Source: CAD feature listing. Evaluate the final solid. Frame: model axes, mm. A direction names the side the tool comes from. Round coordinates to 2 decimals unless told otherwise and drop trailing zeros. Loops run counter-clockwise (first coordinate to the right, second up) from the corner with the lowest first, then second, coordinate; pieces in that order, holes last. Notation, with made-up numbers: M -8,12 L 34,12 A16 ccw 34,43 Z; hole C -6.75,23 d10. An arc over 180 degrees is marked long. Write each question's results on one line, items separated by ' | '. Start each with the question number.
1. Set-up query: faces 5 (the flat face through (-12, 108, -20)), 6 (the flat face through (0, 125, -10)), 7 (the flat face through (10, 1, -124)). Return all of +Z, -Z, +X, -X, +Y, -Y with unobstructed straight access to the full face (end or side cutting, diameter ignored); none if empty.
2. Section C-C on x = -5. Output: boundary loops of the cut face in (y, z), and give its area (3 significant figures).
3. Section A-A on z = -42.5. Output: boundary loops of the cut face in (x, y).
4. Section B-B on y = -23. Output: boundary loops of the cut face in (x, z).
5. Ray query, line 1 (Y direction, x = 1, z = -21.5); line 2 (Z direction, x = -3.75, y = -42); line 3 (Z direction, x = 1.5, y = 52.5). Return the intervals inside material, ascending.
6. Contact query for flat-ended pins moving along their axis: pin 1 Ø22 at (y, z) = (9.5, -0.5) entering from -X; pin 2 Ø12 at (x, z) = (0.5, -51) entering from +Y; pin 3 Ø5.5 at (x, y) = (13.5, -106) entering from -Z. Output: stop coordinate, or through.
7. Draft query along Z for faces 1 (the flat face through (0, 1, -15)), 2 (the flat face through (-15, -108, -5)), 3 (the flat face through (0, 2, 10)), 4 (the flat face through (0, -125, -10)). Return one class per face: released by +Z, released by -Z, zero draft, split by the parting line, or undercut.
8. Section D-D on y = -108. Output: boundary loops of the cut face in (x, z).
from build123d import *

# Parameters (mm, degrees)
F0_W      = 20
F0_H      = 275
F1_DEPTH  = 10
F3_W      = 20
F3_H      = 110
F3_H_2    = 20
F4_DEPTH  = 10
F6_W      = 20
F6_H      = 20
F6_H_2    = 110
F7_DEPTH  = 10
F8_W      = 20
F8_H      = 205
F9_DEPTH  = 10
F10_W     = 5
F10_H     = 220
F11_DEPTH = 15


with BuildPart() as f1:
    # F0 (on Top) → F1 (new body, symmetric)
    with BuildSketch(Plane.XY):
        Rectangle(F0_W, F0_H)
    extrude(amount=F1_DEPTH, both=True)

    # F3 (on offset) → F4 (join)
    with BuildSketch(Plane.XZ.offset(112.5)):
        with Locations((0, -75)):
            Rectangle(F3_W, F3_H)
        with Locations((0, -10)):
            Rectangle(F3_W, F3_H_2)
        Polygon((15, -20), (15, 10), (-15, 10), (-15, -20), (-10, -20), (-10, 0), (10, 0), (10, -20), align=None)
    extrude(amount=-F4_DEPTH)

    # F6 (on offset) → F7 (join)
    with BuildSketch(Plane(origin=(0, 112.5, 0), x_dir=(-1, 0, 0), z_dir=(0, 1, 0))):
        with Locations((0, -10)):
            Rectangle(F6_W, F6_H)
        with Locations((0, -75)):
            Rectangle(F6_W, F6_H_2)
        Polygon((15, -20), (15, 10), (-15, 10), (-15, -20), (-10, -20), (-10, 0), (10, 0), (10, -20), align=None)
    extrude(amount=-F7_DEPTH)

    # F8 (on face) → F9 (join)
    with BuildSketch(Plane(origin=(0, 0, -130), x_dir=(1, 0, 0), z_dir=(0, 0, -1))):
        Rectangle(F8_W, F8_H)
    extrude(amount=-F9_DEPTH)

    # F10 (on Top) → F11 (join)
    with BuildSketch(Plane.XY):
        Rectangle(F10_W, F10_H)
    extrude(amount=-F11_DEPTH)


solid = f1.part
Taken from the geometry:
1) face 5: -Z, -X, +Y, -Y | face 6: -Z, +X, -X, +Y | face 7: -Z, +X, +Y, -Y
2) outline: M -137.5,-10 L -112.5,-10 L -112.5,-130 L 112.5,-130 L 112.5,-10 L 137.5,-10 L 137.5,10 L -137.5,10 Z; hole M -102.5,-120 L 102.5,-120 L 102.5,-10 L -102.5,-10 Z | area: 9,950 mm^2
3) outline: M -10,-112.5 L 10,-112.5 L 10,-102.5 L -10,-102.5 Z; M -10,102.5 L 10,102.5 L 10,112.5 L -10,112.5 Z
4) outline: M -10,-130 L 10,-130 L 10,-120 L -10,-120 Z; M -10,-10 L -2.5,-10 L -2.5,-15 L 2.5,-15 L 2.5,-10 L 10,-10 L 10,10 L -10,10 Z
5) line 1: -112.5 to -102.5, 102.5 to 112.5 | line 2: -130 to -120, -10 to 10 | line 3: -130 to -120, -15 to 10
6) pin 1: x = -10 | pin 2: y = 112.5 | pin 3: z = -20
7) face 1: undercut | face 2: zero draft | face 3: released by +Z | face 4: released by -Z
8) outline: M -15,-20 L -10,-20 L -10,-130 L 10,-130 L 10,-20 L 15,-20 L 15,10 L -15,10 Z
